from build123d import *

# Parameters (mm, degrees)
SKETCH1_W                                  = 24.7396
SKETCH1_H                                  = 37.719
BOSS_EXTRUDE1_DEPTH                        = 4.2418
BOSS_EXTRUDE2_DEPTH                        = 2.9464
MIRROR2_COPY_1_DEPTH                       = 2.9464
SKETCH3_W                                  = 6.985
SKETCH3_H                                  = 31.8262
CUT_EXTRUDE1_DEPTH                         = 1.3462
LPATTERN1_COUNT                            = 3
LPATTERN1_PITCH                            = 7.9502
SKETCH4_R                                  = 1.0668
CUT_EXTRUDE2_DEPTH                         = 40.958840453
SKETCH5_R                                  = 1.9812
CUT_EXTRUDE3_DEPTH                         = 1.524
MIRROR4_AT_THE_SECOND_PLANE_COPY_1_SKETC_R = 1.9812
MIRROR4_AT_THE_SECOND_PLANE_COPY_1_DEPTH   = 1.524
SKETCH6_W                                  = 7.112
SKETCH6_H                                  = 2.8956
CUT_EXTRUDE4_DEPTH                         = 25.218015153
SKETCH7_W                                  = 6.987300404
SKETCH7_H                                  = 1.344727602
CUT_EXTRUDE5_DEPTH                         = 63.5
CHAMFER2_SIZE                              = 1.905
SKETCH8_W                                  = 4.318
SKETCH8_H                                  = 33.909
BOSS_EXTRUDE3_DEPTH                        = 25.4
SKETCH9_R                                  = 1.651
CUT_EXTRUDE6_DEPTH                         = 25.4
FILLET1_R                                  = 10
FILLET2_R                                  = 3.81
LPATTERN4_COUNT                            = 2
LPATTERN4_PITCH                            = 6.35
LPATTERN4_COUNT_DIR2                       = 4
LPATTERN4_PITCH_DIR2                       = 6.35
LPATTERN5_COUNT                            = 2
LPATTERN5_PITCH                            = 6.35
LPATTERN5_COPY_1_SKETCH_R                  = 1.651
LPATTERN5_COPY_1_DEPTH                     = 25.4
LPATTERN5_COPY_2_SKETCH_R                  = 1.651
LPATTERN5_COPY_2_DEPTH                     = 25.4
LPATTERN5_COPY_3_SKETCH_R                  = 1.651
LPATTERN5_COPY_3_DEPTH                     = 25.4
LPATTERN5_COPY_4_SKETCH_R                  = 1.651
LPATTERN5_COPY_4_DEPTH                     = 25.4
LPATTERN5_COPY_5_SKETCH_R                  = 1.651
LPATTERN5_COPY_5_DEPTH                     = 25.4
LPATTERN5_COPY_6_SKETCH_R                  = 1.651
LPATTERN5_COPY_6_DEPTH                     = 25.4
LPATTERN5_COPY_7_SKETCH_R                  = 1.651
LPATTERN5_COPY_7_DEPTH                     = 25.4
CUT_EXTRUDE7_DEPTH                         = 25.4


with BuildPart() as part:
    # Sketch1 → Boss-Extrude1 (new body)
    with BuildSketch(Plane(origin=(0, 0, 0), x_dir=(1, 0, 0), z_dir=(0, 1, 0))):
        Rectangle(SKETCH1_W, SKETCH1_H)
    extrude(amount=BOSS_EXTRUDE1_DEPTH)

    # Sketch2 → Boss-Extrude2 (add)
    with BuildSketch(Plane(origin=(0, 0, -18.8595), x_dir=(-1, 0, 0), z_dir=(0, 0, -1))):
        Polygon((-12.3698, -1.7018), (-12.3698, 4.2418), (-3.6068, 4.2418), (-3.6068, -1.7018), (-6.4643, -4.579739869), (-9.5123, -4.579739869), align=None)
    boss_extrude2 = extrude(amount=-BOSS_EXTRUDE2_DEPTH)

    # Mirror1: Boss-Extrude2 across plane
    add(boss_extrude2.mirror(Plane(origin=(0, 0, 0), x_dir=(0, 0, 1), z_dir=(1, 0, 0))))

    # Mirror2: Boss-Extrude2 across plane
    add(boss_extrude2.mirror(Plane.XY))

    # Mirror2 copy 1 sketch → Mirror2 copy 1 (add)
    with BuildSketch(Plane.XY.offset(18.8595)):
        Polygon((-12.3698, -1.7018), (-12.3698, 4.2418), (-3.6068, 4.2418), (-3.6068, -1.7018), (-6.4643, -4.579739869), (-9.5123, -4.579739869), align=None)
    extrude(amount=-MIRROR2_COPY_1_DEPTH)

    # Sketch3 → Cut-Extrude1 (cut)
    with BuildSketch(Plane.XZ):
        with Locations((-7.8613, 0)):
            Rectangle(SKETCH3_W, SKETCH3_H)
    cut_extrude1 = extrude(amount=-CUT_EXTRUDE1_DEPTH, mode=Mode.SUBTRACT)

    # LPattern1: Cut-Extrude1 ×3
    with Locations(*[(i * LPATTERN1_PITCH, 0, 0) for i in range(1, LPATTERN1_COUNT)]):
        add(cut_extrude1, mode=Mode.SUBTRACT)

    # Sketch4 → Cut-Extrude2 (cut, symmetric)
    with BuildSketch(Plane(origin=(0, 0, -18.8595), x_dir=(-1, 0, 0), z_dir=(0, 0, -1))):
        with Locations((-7.9883, -1.201539869)):
            Circle(SKETCH4_R)
    cut_extrude2 = extrude(amount=CUT_EXTRUDE2_DEPTH, both=True, mode=Mode.SUBTRACT)

    # Mirror3: Cut-Extrude2 across plane
    add(cut_extrude2.mirror(Plane(origin=(0, 0, 0), x_dir=(0, 0, 1), z_dir=(1, 0, 0))), mode=Mode.SUBTRACT)

    # Sketch5 → Cut-Extrude3 (cut)
    with BuildSketch(Plane(origin=(0, 0, -18.8595), x_dir=(-1, 0, 0), z_dir=(0, 0, -1))):
        with Locations((-7.9883, -1.201539869)):
            Circle(SKETCH5_R)
    cut_extrude3 = extrude(amount=-CUT_EXTRUDE3_DEPTH, mode=Mode.SUBTRACT)

    # Mirror4: Cut-Extrude3 across plane
    add(cut_extrude3.mirror(Plane.XY), mode=Mode.SUBTRACT)

    # Mirror4 at the second plane: Cut-Extrude3 across plane
    add(cut_extrude3.mirror(Plane(origin=(0, 0, 0), x_dir=(0, 0, 1), z_dir=(1, 0, 0))), mode=Mode.SUBTRACT)

    # Mirror4 at the second plane copy 1 sketc → Mirror4 at the second plane copy 1 (cut)
    with BuildSketch(Plane.XY.offset(18.8595)):
        with Locations((-7.9883, -1.201539869)):
            Circle(MIRROR4_AT_THE_SECOND_PLANE_COPY_1_SKETC_R)
    extrude(amount=-MIRROR4_AT_THE_SECOND_PLANE_COPY_1_DEPTH, mode=Mode.SUBTRACT)

    # Sketch6 → Cut-Extrude4 (cut, through all)
    with BuildSketch(Plane(origin=(0, 4.2418, 0), x_dir=(1, 0, 0), z_dir=(0, 1, 0))):
        with Locations((-0.0254, 17.4117)):
            Rectangle(SKETCH6_W, SKETCH6_H)
    cut_extrude4 = extrude(amount=-CUT_EXTRUDE4_DEPTH, mode=Mode.SUBTRACT)

    # Mirror5: Cut-Extrude4 across plane
    add(cut_extrude4.mirror(Plane.XY), mode=Mode.SUBTRACT)

    # Sketch7 → Cut-Extrude5 (cut, symmetric)
    with BuildSketch(Plane(origin=(0, 0, 15.9131), x_dir=(-1, 0, 0), z_dir=(0, 0, -1))):
        with Locations((-0.083466761, 0.672363801)):
            Rectangle(SKETCH7_W, SKETCH7_H)
    extrude(amount=CUT_EXTRUDE5_DEPTH, both=True, mode=Mode.SUBTRACT)

    # Chamfer2
    chamfer2_edges = [part.edges().sort_by_distance(p)[0] for p in [
        (7.9502, 4.2418, -18.8595),
        (-7.9756, 4.2418, -18.8595),
        (7.9502, 4.2418, 18.8595),
        (-7.9756, 4.2418, 18.8595),
    ]]
    chamfer(chamfer2_edges, length=CHAMFER2_SIZE)

    # Sketch8 → Boss-Extrude3 (add)
    with BuildSketch(Plane(origin=(0, 4.2418, 0), x_dir=(1, 0, 0), z_dir=(0, 1, 0))):
        with Locations((-10.2108, 0)):
            Rectangle(SKETCH8_W, SKETCH8_H)
    extrude(amount=BOSS_EXTRUDE3_DEPTH)

    # Sketch9 → Cut-Extrude6 (cut)
    with BuildSketch(Plane(origin=(-8.0518, 0, 0), x_dir=(0, 0, -1), z_dir=(1, 0, 0))):
        with Locations((9.9695, 16.51)):
            Circle(SKETCH9_R)
    cut_extrude6 = extrude(amount=-CUT_EXTRUDE6_DEPTH, mode=Mode.SUBTRACT)

    # Fillet1
    fillet1_edges = [part.edges().sort_by_distance(p)[0] for p in [
        (-10.2108, 29.6418, 16.9545),
        (-10.2108, 29.6418, -16.9545),
    ]]
    fillet(fillet1_edges, radius=FILLET1_R)

    # Fillet2
    fillet2_edges = [part.edges().sort_by_distance(p)[0] for p in [
        (-8.0518, 4.2418, 0),
    ]]
    fillet(fillet2_edges, radius=FILLET2_R)

    # LPattern4: Cut-Extrude6 2 × 4
    with Locations(*[(0, -i * LPATTERN4_PITCH, j * LPATTERN4_PITCH_DIR2) for i in range(LPATTERN4_COUNT) for j in range(LPATTERN4_COUNT_DIR2) if (i, j) != (0, 0)]):
        add(cut_extrude6, mode=Mode.SUBTRACT)

    # LPattern5: Cut-Extrude6 ×2
    with Locations(*[(0, i * LPATTERN5_PITCH, 0) for i in range(1, LPATTERN5_COUNT)]):
        add(cut_extrude6, mode=Mode.SUBTRACT)

    # LPattern5 copy 1 sketch → LPattern5 copy 1 (cut)
    with BuildSketch(Plane(origin=(-8.0518, 6.35, 6.35), x_dir=(0, 0, -1), z_dir=(1, 0, 0))):
        with Locations((9.9695, 16.51)):
            Circle(LPATTERN5_COPY_1_SKETCH_R)
    extrude(amount=-LPATTERN5_COPY_1_DEPTH, mode=Mode.SUBTRACT)

    # LPattern5 copy 2 sketch → LPattern5 copy 2 (cut)
    with BuildSketch(Plane(origin=(-8.0518, 6.35, 12.7), x_dir=(0, 0, -1), z_dir=(1, 0, 0))):
        with Locations((9.9695, 16.51)):
            Circle(LPATTERN5_COPY_2_SKETCH_R)
    extrude(amount=-LPATTERN5_COPY_2_DEPTH, mode=Mode.SUBTRACT)

    # LPattern5 copy 3 sketch → LPattern5 copy 3 (cut)
    with BuildSketch(Plane(origin=(-8.0518, 6.35, 19.05), x_dir=(0, 0, -1), z_dir=(1, 0, 0))):
        with Locations((9.9695, 16.51)):
            Circle(LPATTERN5_COPY_3_SKETCH_R)
    extrude(amount=-LPATTERN5_COPY_3_DEPTH, mode=Mode.SUBTRACT)

    # LPattern5 copy 4 sketch → LPattern5 copy 4 (cut)
    with BuildSketch(Plane(origin=(-8.0518, 0, 0), x_dir=(0, 0, -1), z_dir=(1, 0, 0))):
        with Locations((9.9695, 16.51)):
            Circle(LPATTERN5_COPY_4_SKETCH_R)
    extrude(amount=-LPATTERN5_COPY_4_DEPTH, mode=Mode.SUBTRACT)

    # LPattern5 copy 5 sketch → LPattern5 copy 5 (cut)
    with BuildSketch(Plane(origin=(-8.0518, 0, 6.35), x_dir=(0, 0, -1), z_dir=(1, 0, 0))):
        with Locations((9.9695, 16.51)):
            Circle(LPATTERN5_COPY_5_SKETCH_R)
    extrude(amount=-LPATTERN5_COPY_5_DEPTH, mode=Mode.SUBTRACT)

    # LPattern5 copy 6 sketch → LPattern5 copy 6 (cut)
    with BuildSketch(Plane(origin=(-8.0518, 0, 12.7), x_dir=(0, 0, -1), z_dir=(1, 0, 0))):
        with Locations((9.9695, 16.51)):
            Circle(LPATTERN5_COPY_6_SKETCH_R)
    extrude(amount=-LPATTERN5_COPY_6_DEPTH, mode=Mode.SUBTRACT)

    # LPattern5 copy 7 sketch → LPattern5 copy 7 (cut)
    with BuildSketch(Plane(origin=(-8.0518, 0, 19.05), x_dir=(0, 0, -1), z_dir=(1, 0, 0))):
        with Locations((9.9695, 16.51)):
            Circle(LPATTERN5_COPY_7_SKETCH_R)
    extrude(amount=-LPATTERN5_COPY_7_DEPTH, mode=Mode.SUBTRACT)

    # Sketch10 → Cut-Extrude7 (cut)
    with BuildSketch(Plane.ZY.offset(12.3698)):
        Polygon((16.9545, 18.479805683), (13.467820237, 16.466770183), (16.9545, 14.453734683), align=None)
    extrude(amount=-CUT_EXTRUDE7_DEPTH, mode=Mode.SUBTRACT)


solid = part.part
Geometry: final body of the model. Coordinates: model frame, mm. A direction names the side the tool comes from. Round coordinates to 2 decimals unless told otherwise and drop trailing zeros. Loops run counter-clockwise (first coordinate to the right, second up) from the corner with the lowest first, then second, coordinate; pieces in that order, holes last. Notation, with made-up numbers: M -17.75,29.5 L 20.25,29.5 A21 ccw 20.25,41.5 Z; hole C 26,60 d7. An arc over 180 degrees is marked long. Put each result on its own line as item: value. Start each with the question number.
(1) Set-up query: faces 1 (the face through (-3.581, 2, -17)), 2 (the face through (-10, 9, 16.954)), 3 (the face through (-10.241, 15.474, 15.187)), 4 (the face through (-3.41, 1, 0)). Return all of +Z, -Z, +X, -X, +Y, -Y with unobstructed straight access to the full face (end or side cutting, diameter ignored); none if empty.
(2) Section query A-A (y = 10.16). Return loops of the section in (x, z), then the cut area to 3 significant figures.
(3) Material intervals for line 1 along X through (y, z) = (0.5, -13); line 2 along Z through (x, y) = (6, 0.5); line 3 along Y through (x, z) = (-10, -9), sorted ascending. Write a range as [from, to].
(4) Section query B-B (z = -2.5). State how many separate pieces and enclosed holes the cut face has, then the cut area to 3 significant figures.
(5) Contact query for flat-ended pins moving along their axis: pin 1 Ø0.7 at (x, z) = (12, 4) entering from -Y; pin 2 Ø5 at (y, z) = (20.5, -5.5) entering from +X; pin 3 Ø1.8 at (x, y) = (7.5, -2) entering from +Z; pin 4 Ø3 at (y, z) = (16.51, -9.97) entering from -X. Output: stop coordinate, or through.
(6) Draft query along Z for faces 5 (the face through (-11.354, 1, 0)), 6 (the face through (-10.92, -3.16, 17.41)), 7 (the face through (-10.24, 17.49, 15.24)), 8 (the face through (-10.181, 11.276, 10.297)). Return one class per face: +Z half, -Z half, draft (parallel to the pull), parting line (faces both ways), or undercut.
Findings below:
1. face 1: -Z, +Y, -Y
1. face 2: +Z, +X, -X, +Y
1. face 3: +Z, +X, -X
1. face 4: +Z, -Z, -Y
2. outline: M -12.37,-16.95 L -8.05,-16.95 L -8.05,-11.62 L -12.37,-11.62 Z; M -12.37,-8.32 L -8.05,-8.32 L -8.05,-5.27 L -12.37,-5.27 Z; M -12.37,-1.97 L -8.05,-1.97 L -8.05,1.08 L -12.37,1.08 Z; M -12.37,4.38 L -8.05,4.38 L -8.05,7.43 L -12.37,7.43 Z; M -12.37,10.73 L -8.05,10.73 L -8.05,16.95 L -12.37,16.95 Z
2. area: 89.4 mm2
3. line 1: x = [-12.37, -11.35], [-4.37, -3.41], [3.58, 4.55], [11.53, 12.37]
3. line 2: z = [-18.86, -15.91], [15.91, 18.86]
3. line 3: y = [1.35, 8.82], [11.5, 15.17], [17.85, 21.52], [24.2, 29.43]
4. separate pieces: 4
4. enclosed holes: 0
4. area: 158 mm2
5. pin 1: stops at y = 0
5. pin 2: stops at x = -8.05
5. pin 3: stops at z = 17.34
5. pin 4: passes through
6. face 5: undercut
6. face 6: draft
6. face 7: +Z half
6. face 8: undercut
